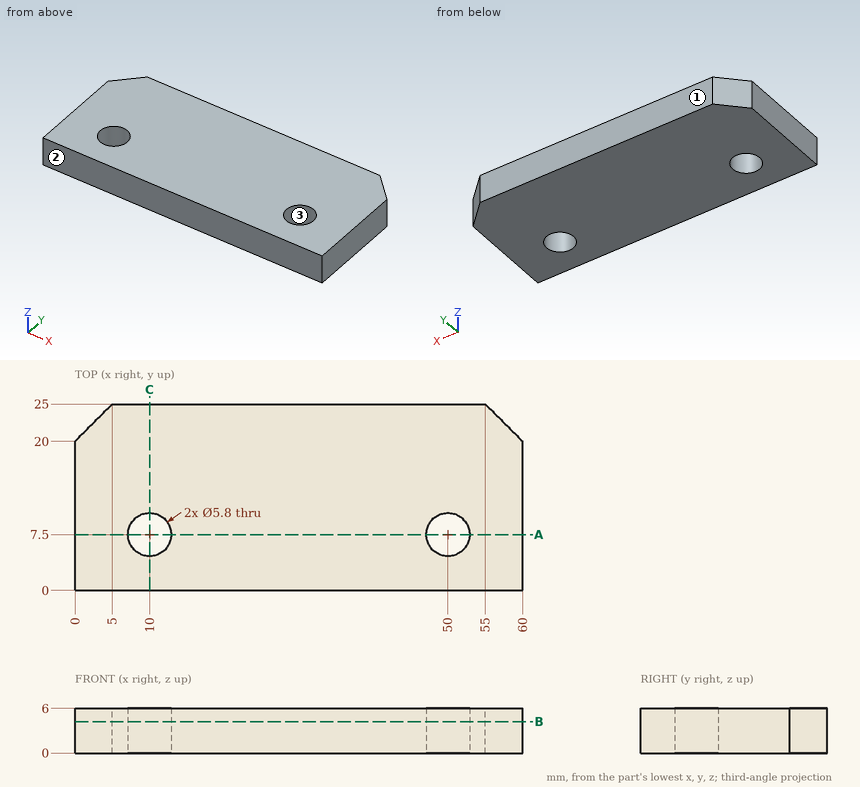
Drawing for the job (mm, zero at the part's lowest x, y, z). Round coordinates to 2 decimals unless told otherwise and drop trailing zeros. Loops run counter-clockwise (first coordinate to the right, second up) from the corner with the lowest first, then second, coordinate; pieces in that order, holes last. Notation, with made-up numbers: (16.25, 84.25) -> (65.25, 84.25) arc R11 ccw to (65.25, 91.25) -> close; hole circle Ø10 at (33, 87). An arc over 180 degrees is marked (long way). Answer in a Markdown table with one row per item.
Item 1: Saw through at A-A (y = 7.5). Write the cut outline in (x, z).
Answers below:
| item | result |
|---|---|
| outline | (0, 0) -> (7.1, 0) -> (7.1, 6) -> (0, 6) -> close; (12.9, 0) -> (47.1, 0) -> (47.1, 6) -> (12.9, 6) -> close; (52.9, 0) -> (60, 0) -> (60, 6) -> (52.9, 6) -> close |
Item 2: Saw through at B-B (z = 4.25). Write the cut outline in (x, y), and give its area (3 significant figures).
Answers below:
| item | result |
|---|---|
| outline | (0, 0) -> (60, 0) -> (60, 20) -> (55, 25) -> (5, 25) -> (0, 20) -> close; hole circle Ø5.8 at (10, 7.5); hole circle Ø5.8 at (50, 7.5) |
| area | 1,420 mm² |
Item 3: Mould opens along Y. For the marked faces 1, 2 and 3 say: +Y half, -Y half, draft (parallel to the pull), parting line (faces both ways), or undercut.
Answers below:
| item | result |
|---|---|
| face 1 | +Y half |
| face 2 | -Y half |
| face 3 | undercut |
Item 4: Saw through at C-C (x = 10). Write the cut outline in (y, z).
Answers below:
| item | result |
|---|---|
| outline | (0, 0) -> (4.6, 0) -> (4.6, 6) -> (0, 6) -> close; (10.4, 0) -> (25, 0) -> (25, 6) -> (10.4, 6) -> close |
Item 5: Drill centre lines: L1, parallel to Y at x = 10, z = 1.35; L2, parallel to X at y = 8.5, z = 3.85; L3, parallel to Y at x = 49, z = 1.3. Where is each one in solid material? Low to high. Write a range as [from, to].
Answers below:
| item | result |
|---|---|
| L1 | y = [0, 4.6], [10.4, 25] |
| L2 | x = [0, 7.28], [12.72, 47.28], [52.72, 60] |
| L3 | y = [0, 4.78], [10.22, 25] |
Item 6: Pin check, flat tip, straight feed: pin 1 (3 mm diameter, centred on x = 16.5, z = 4.5, fed in from -Y). Stop position of the tip, or through.
Answers below:
| item | result |
|---|---|
| pin 1 | stops at y = 0 |
